For this review, take the finished solid that the model builds, in its own axes (mm). A direction names the side the tool comes from. Coordinates: 2 decimals unless noted, no trailing zeros. Write each loop counter-clockwise with the first axis right and the second up, starting at its lowest first coordinate (ties: lowest second). Pieces come first, ordered by that corner, then holes. Notation, with made-up numbers: (29, -37) -> (41, -37) arc R20 cw to (41, -4) -> close; hole circle Ø8 at (32, -3.5). An arc over 180 degrees is marked (long way). One line per item, written item: value. Start each with the question number.
1) Mouldability with a two-part tool opening along X and no side actions: class faces 1 (the flat face through (42, 4, 12)), 2 (the flat face through (35, 0, 17)), 3 (the flat face through (32, 36, 33)) as released by +X, released by -X, zero draft, split by the parting line, or undercut.
2) Add section D-D (y = 22.5). State the section outline as (x, z) points, and give its area (3 significant figures).
3) For probe 1 along X at (y, z) = (21, 25); probe 2 along Y at (x, z) = (15.5, -1); probe 3 along Y at (x, z) = (34, 9.5), list the stretches that pass through material, from the lowest coordinate up. Write a range as from..to.
4) Add section C-C (x = 42.5). State the section outline as (y, z) points.
5) Add section B-B (y = 11). State the section outline as (x, z) points.
6) Machinability: for faces 4 (the flat face through (49, 38, 21)), 5 (the flat face through (42, 54, 53)), 6 (the flat face through (42, 39, 51)), which of the approach directions +Z, -Z, +X, -X, +Y, -Y give a long, thin tool a straight path to every point of the face, cutting with its end or side? Answer none if there is none.
7) Add section A-A (z = 41). State the section outline as (x, y) points.
8) For pin 1 Ø1.5 at (y, z) = (16, 42) entering from -X; pin 2 Ø3.5 at (x, z) = (39, 43.5) entering from -Y; pin 3 Ø12 at (y, z) = (13.5, 28) entering from +X; pin 4 Ø6 at (x, y) = (26.5, 14.5) entering from +Z, all flat-tipped, find the tip position at first contact; note any pin that passes through.
Autodesk Inventor part; units mm, degrees
ref_plane "YZ Plane" through (0, 0, 0) normal (1, 0, 0) x (0, 1, 0)
ref_plane "XY Plane" through (0, 0, 0) normal (0, 0, 1) x (1, 0, 0)
sketch "Skizze1" plane through (0, 0, 0) normal (0, 0, 1) x (1, 0, 0)
  line L0 (-60, 0) -> (60, 0)
  line L1 (60, 0) -> (60, 20)
  line L2 (60, 20) -> (-60, 20)
  line L3 (-60, 20) -> (-60, 0)
  point P0 (0, 0)
  dimension "d0" = 120
  dimension "d1" = 20
extrude "Extrusion1" add sketch "Skizze1" against normal blind 4
sketch "Skizze2" plane through (0, 0, 0) normal (0, 1, 0) x (-1, 0, 0)
  line L0 (-60, 0) -> (60, 0)
  line L1 (-52, 0) -> (-32, 0)
  line L2 (-32, 0) -> (-32, 55)
  line L3 (-32, 55) -> (-52, 55)
  line L4 (-52, 55) -> (-52, 0)
  point P0 (0, 0)
  dimension "d17" = 20
  dimension "d18" = 55
extrude "Extrusion2" add sketch "Skizze2" along normal blind 4
sketch "Skizze8" plane through (0, 4, 0) normal (0, 1, 0) x (1, 0, 0)
  line L0 (52, -55) -> (52, 0)
  line L1 (32, -55) -> (52, -55)
  line L2 (52, -55) -> (52, -51)
  line L3 (52, -51) -> (32, -51)
  line L4 (32, -51) -> (32, -55)
  point P0 (0, 0)
extrude "Extrusion7" add sketch "Skizze8" along normal blind 50
sketch "Skizze9" plane through (0, 4, 0) normal (0, 1, 0) x (1, 0, 0)
  line L0 (32, 0) -> (32, -51)
  line L1 (32, -51) -> (36, -51)
  line L2 (36, -51) -> (36, -31)
  line L3 (36, -31) -> (32, -31)
  line L4 (32, -31) -> (32, -51)
  line L5 (52, -51) -> (48, -51)
  line L6 (48, -51) -> (48, -31)
  line L7 (48, -31) -> (52, -31)
  line L8 (52, -31) -> (52, -51)
  point P0 (0, 0)
extrude "Extrusion8" add sketch "Skizze9" along normal blind 65
sketch "Skizze10" plane through (48, 4, 51) normal (0, 0, -1) x (-1, 0, 0)
  point P0 (48, -4)
sketch "Skizze11" plane through (0, 4, 0) normal (0, 1, 0) x (1, 0, 0)
  line L0 (48, -51) -> (36, -51)
  line L1 (36, -31) -> (32, -31)
  line L2 (48, -51) -> (36, -51)
  line L3 (36, -51) -> (36, -31)
  line L4 (36, -31) -> (48, -31)
  line L5 (48, -31) -> (48, -51)
  point P0 (0, 0)
extrude "Extrusion9" add sketch "Skizze11" along normal blind 20
ref_plane "Arbeitsebene1" through (0, 69, 0) normal (0, 1, 0) x (-1, 0, 0)
sketch "Skizze12" plane through (0, 69, 0) normal (0, 1, 0) x (-1, 0, 0)
  line L0 (-32, 0) -> (-32, 55)
  line L1 (-52, 55) -> (-32, 55)
  line L2 (-32, 55) -> (-32, 25)
  line L3 (-32, 25) -> (-52, 25)
  line L4 (-52, 25) -> (-52, 55)
  point P0 (0, 0)
extrude "Extrusion10" add sketch "Skizze12" along normal blind 4
sketch "Skizze13" plane through (0, 54, 0) normal (0, 1, 0) x (1, 0, 0)
  point P0 (0, 0)
sketch "Skizze14" plane through (0, 54, 0) normal (0, 1, 0) x (1, 0, 0)
  line L0 (52, -55) -> (52, -25)
  line L1 (48, -31) -> (48, -51)
  line L2 (52, -55) -> (48, -55)
  line L3 (48, -55) -> (48, -51)
  line L4 (48, -51) -> (52, -51)
  line L5 (52, -51) -> (52, -55)
  line L6 (32, -55) -> (36, -55)
  line L7 (36, -55) -> (36, -51)
  line L8 (36, -51) -> (32, -51)
  line L9 (32, -51) -> (32, -55)
  point P0 (0, 0)
extrude "Extrusion11" add sketch "Skizze14" along normal blind 15
sketch "Skizze15" plane through (0, 69, 0) normal (0, 1, 0) x (-1, 0, 0)
  line L0 (-52, 25) -> (-32, 25)
  line L1 (-52, 31) -> (-52, 0)
  line L2 (-32, 25) -> (-52, 25)
  line L3 (-52, 25) -> (-52, 21)
  line L4 (-52, 21) -> (-32, 21)
  line L5 (-32, 21) -> (-32, 25)
  point P0 (0, 0)
extrude "Extrusion12" add sketch "Skizze15" along normal blind 4
sketch "Skizze16" plane through (0, 4, 0) normal (0, 1, 0) x (1, 0, 0)
  line L0 (52, -21) -> (32, -21)
  line L1 (52, -31) -> (48, -31)
  line L2 (52, -21) -> (48, -21)
  line L3 (48, -21) -> (48, -31)
  line L4 (48, -31) -> (52, -31)
  line L5 (52, -31) -> (52, -21)
  line L6 (32, -21) -> (32, -55)
  line L7 (36, -31) -> (32, -31)
  line L8 (32, -21) -> (36, -21)
  line L9 (36, -21) -> (36, -31)
  line L10 (36, -31) -> (32, -31)
  line L11 (32, -31) -> (32, -21)
  point P0 (0, 0)
extrude "Extrusion13" add sketch "Skizze16" along normal blind 65
properties part number "Drehmomentstütze"
Numbers:
1. face 1: undercut
1. face 2: zero draft
1. face 3: released by -X
2. outline: (32, 21) -> (36, 21) -> (36, 31) -> (48, 31) -> (48, 21) -> (52, 21) -> (52, 55) -> (32, 55) -> close
2. area: 560 mm²
3. probe 1: 32..36, 48..52
3. probe 2: 0..20
3. probe 3: 0..4
4. outline: (0, -4) -> (20, -4) -> (20, 0) -> (4, 0) -> (4, 31) -> (24, 31) -> (24, 51) -> (54, 51) -> (54, 55) -> (0, 55) -> close; (69, 21) -> (73, 21) -> (73, 55) -> (69, 55) -> close
5. outline: (-60, -4) -> (60, -4) -> (60, 0) -> (-60, 0) -> close; (32, 21) -> (36, 21) -> (36, 31) -> (48, 31) -> (48, 21) -> (52, 21) -> (52, 55) -> (32, 55) -> close
6. face 4: +X, -X, +Y
6. face 5: +Z, -Z
6. face 6: -Z
7. outline: (32, 0) -> (52, 0) -> (52, 73) -> (32, 73) -> close; hole (36, 24) -> (48, 24) -> (48, 69) -> (36, 69) -> close
8. pin 1: x = 32
8. pin 2: y = 0
8. pin 3: x = 52
8. pin 4: z = 0
